Read the model definition and answer for the solid it produces. Units are mm, in the model's axes. A direction names the side the tool comes from. Coordinates: 2 decimals unless noted, no trailing zeros. Write each loop counter-clockwise with the first axis right and the second up, starting at its lowest first coordinate (ties: lowest second). Pieces come first, ordered by that corner, then holes.
Item 1: A tool of negligible diameter and unlimited length cuts with its end or side. For faces 4 (the face through (32.5, 17, 22)), 5 (the face through (0, -35, 20)), from which of +Z, -Z, +X, -X, +Y, -Y can it reach the whole face along a straight path? Write none if from no direction.
Item 2: Determine the mould class of faces 1 (the face through (0, 35, 20)), 2 (the face through (0, 0, 0)), 3 (the face through (17, 17, 5)) for opening direction Y: released by +Y, released by -Y, zero draft, split by the parting line, or undercut.
Item 3: Section A-A (z = 12) is taken. Give the vertices of the cut face in (x, y), then the cut area to 3 significant figures.
Item 4: Section B-B (x = -14.5) is taken. Give the vertices of the cut face in (y, z).
Item 5: Straight lines are drawn through the part: probe 1 along Y at (x, z) = (-18, 16.5); probe 2 along Z at (x, y) = (-12.5, -6). For each, find the intervals that lie inside material, in ascending order.
Item 6: Each of these flat-tipped pins is pushed along its axis until it touches: P1, Ø2, axis at x = -6.5, y = 27.5, coming from the -Z side; P2, Ø9, axis at x = -24, y = -17, coming from the +Z side. Where does it stop, or does it pass through?
from build123d import *

# Parameters (mm, degrees)
F0_W     = 70
F0_H     = 70
F0_W_2   = 30.75
F0_H_2   = 30.75
F1_DEPTH = 40
F2_DEPTH = 5


with BuildPart() as f1:
    # F0 (on Top) → F1 (new body)
    with BuildSketch(Plane.XY):
        Rectangle(F0_W, F0_H)
        with Locations((-17.125, -17.125)):
            Rectangle(F0_W_2, F0_H_2, mode=Mode.SUBTRACT)
        with Locations((17.125, -17.125)):
            Rectangle(F0_W_2, F0_H_2, mode=Mode.SUBTRACT)
        with Locations((-17.125, 17.125)):
            Rectangle(F0_W_2, F0_H_2, mode=Mode.SUBTRACT)
        with Locations((17.125, 17.125)):
            Rectangle(F0_W_2, F0_H_2, mode=Mode.SUBTRACT)
    extrude(amount=F1_DEPTH)

    # F0 (on Top) → F2 (join)
    with BuildSketch(Plane.XY):
        with Locations((17.125, 17.125)):
            Rectangle(F0_W_2, F0_H_2)
        with Locations((17.125, -17.125)):
            Rectangle(F0_W_2, F0_H_2)
        with Locations((-17.125, -17.125)):
            Rectangle(F0_W_2, F0_H_2)
        with Locations((-17.125, 17.125)):
            Rectangle(F0_W_2, F0_H_2)
    extrude(amount=F2_DEPTH)


solid = f1.part
Established:
1. face 4: +Z
1. face 5: +Z, -Z, +X, -X, -Y
2. face 1: released by +Y
2. face 2: zero draft
2. face 3: undercut
3. outline: (-35, -35) - (35, -35) - (35, 35) - (-35, 35) - close; hole (-32.5, -32.5) - (-1.75, -32.5) - (-1.75, -1.75) - (-32.5, -1.75) - close; hole (-32.5, 1.75) - (-1.75, 1.75) - (-1.75, 32.5) - (-32.5, 32.5) - close; hole (1.75, -32.5) - (32.5, -32.5) - (32.5, -1.75) - (1.75, -1.75) - close; hole (1.75, 1.75) - (32.5, 1.75) - (32.5, 32.5) - (1.75, 32.5) - close
3. area: 1,120 mm2
4. outline: (-35, 0) - (35, 0) - (35, 40) - (32.5, 40) - (32.5, 5) - (1.75, 5) - (1.75, 40) - (-1.75, 40) - (-1.75, 5) - (-32.5, 5) - (-32.5, 40) - (-35, 40) - close
5. probe 1: y = -35 to -32.5, -1.75 to 1.75, 32.5 to 35
5. probe 2: z = 0 to 5
6. P1: stops at z = 0
6. P2: stops at z = 5
